Here's the drawing with two shaded views (mm, measured from the low corner). I have some questions. A direction names the side the tool comes from. Coordinates: 2 decimals unless noted, no trailing zeros. Write each loop counter-clockwise with the first axis right and the second up, starting at its lowest first coordinate (ties: lowest second). Pieces come first, ordered by that corner, then holes. Notation, with made-up numbers: M 51,-5.5 L 109,-5.5 A15 cw 109,7.5 Z; hole C -30,88 d6. An arc over 180 degrees is marked long. Use one line per item in the form item = value. Start each with the question number.
1. I'm going to push flat-ended pins straight in: pin 1 Ø7 at (x, y) = (10, 10) entering from +Z; pin 2 Ø1.5 at (x, z) = (14, 7) entering from -Y; pin 3 Ø1.5 at (x, y) = (7, 10.5) entering from -Z; pin 4 Ø1 at (x, z) = (10, 1.5) entering from +Y. Where does each tip first touch, or does it pass through?
2. On a 3-axis mill with a long thin cutter (end or side, diameter ignored), from which of +Z, -Z, +X, -X, +Y, -Y can I reach the whole of each face in a straight line? I mean the marked faces 1, 2 and 3. Say none if no direction works.
3. Please list where these lines run through material, in increasing order: line 1 along Z through (x, y) = (15.5, 12.75); line 2 along Z through (x, y) = (4.75, 12); line 3 along X through (y, z) = (12.75, 1.75). Write a range as [from, to].
4. I want a section at C-C, the plane z = 3. List the corners of the cut face in (x, y) for me, plus the area to 3 significant figures.
5. I want a section at D-D, the plane z = 5.5. List the corners of the cut face in (x, y) for me, plus the area to 3 significant figures.
6. I want a section at A-A, the plane y = 10. List the corners of the cut face in (x, z) for me, plus the area to 4 significant figures.
7. Thinking about a two-plate mould opening in X: for the marked faces 4, 5, 6 and 7, which applies, released by +X, released by -X, zero draft, split by the parting line, or undercut?
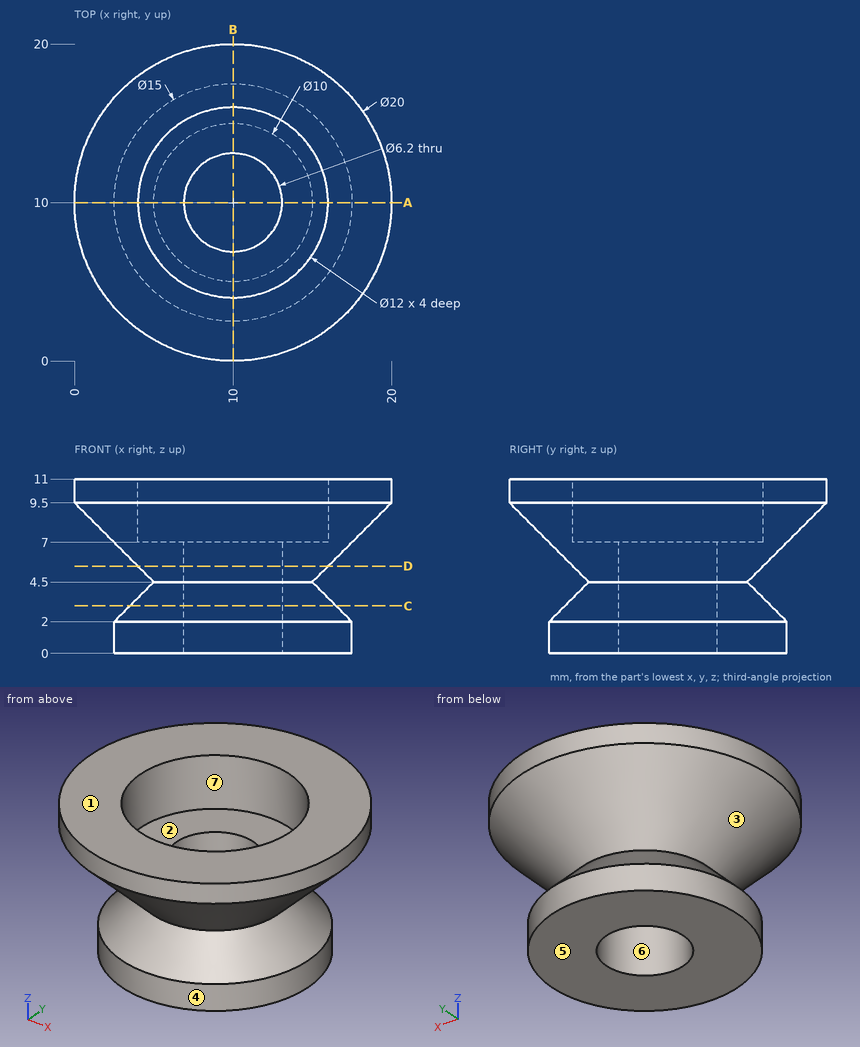
Answer list:
q1.pin_1 = 7
q1.pin_2 = 2.7
q1.pin_3 = 0
q1.pin_4 = 17.5
q2.face_1 = +Z, +X, -X, +Y, -Y
q2.face_2 = +Z
q2.face_3 = none
q3.line_1 = [0, 3.35], [5.65, 11]
q3.line_2 = [0, 3.88], [5.12, 7]
q3.line_3 = [3.02, 8.57], [11.43, 16.98]
q4.outline = C 10,10 d13; hole C 10,10 d6.2
q4.area = 103 mm²
q5.outline = C 10,10 d12; hole C 10,10 d6.2
q5.area = 82.9 mm²
q6.outline = M 0,9.5 L 5,4.5 L 2.5,2 L 2.5,0 L 6.9,0 L 6.9,7 L 4,7 L 4,11 L 0,11 Z; M 13.1,0 L 17.5,0 L 17.5,2 L 15,4.5 L 20,9.5 L 20,11 L 16,11 L 16,7 L 13.1,7 Z
q6.area = 74.85 mm²
q7.face_4 = split by the parting line
q7.face_5 = zero draft
q7.face_6 = undercut
q7.face_7 = undercut
